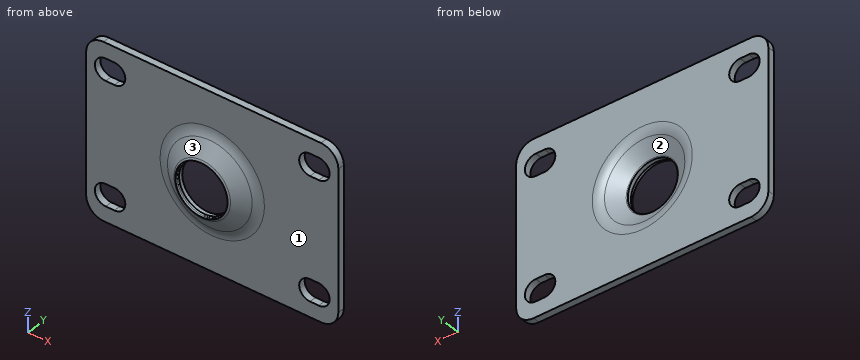
from build123d import *

# Parameters (mm, degrees)
SK_PLATE_OUTLINE_SLOTS_R = 19.05
EXT_PLATE_DEPTH          = 2.54


with BuildPart() as part:
    # Sk_pressed_centre → Rev_pressed_centre (revolve)
    with BuildSketch(Plane.XY, mode=Mode.PRIVATE) as rev_pressed_centre_sk:
        with BuildLine():
            Line((19.304, 69.85), (18.2626, 69.85))
            ThreePointArc((18.2626, 69.85), (16.381490046, 69.564975304), (14.669516, 68.73494))
            Line((14.669516, 68.73494), (9.54024, 65.2145))
            ThreePointArc((9.54024, 65.2145), (9.341458064, 65.091180356), (9.1313, 64.98844))
            Line((9.1313, 64.98844), (9.1313, 63.5508))
            Line((9.1313, 63.5508), (9.1567, 63.5508))
            ThreePointArc((9.1567, 63.5508), (9.426107684, 63.439207684), (9.5377, 63.1698))
            Line((9.5377, 63.1698), (9.5377, 62.31382))
            ThreePointArc((9.5377, 62.31382), (9.947965238, 62.460661275), (10.32764, 62.6745))
            Line((10.32764, 62.6745), (15.45717, 66.19494))
            ThreePointArc((15.45717, 66.19494), (17.169221611, 67.02429691), (19.05, 67.31))
            Line((19.05, 67.31), (19.304, 67.31))
            Line((19.304, 67.31), (19.304, 69.85))
        make_face()
    revolve(rev_pressed_centre_sk.sketch.rotate(Axis((0, -25.4, 0), (0, 1, 0)), 90), axis=Axis((0, -25.4, 0), (0, 1, 0)))

    # Sk_plate_outline_slots → Ext_plate (add)
    with BuildSketch(Plane(origin=(0, 67.31, 0), x_dir=(1, 0, 0), z_dir=(0, 1, 0))):
        with BuildLine():
            Line((-39.6875, 31.75), (39.6875, 31.75))
            ThreePointArc((39.6875, 31.75), (44.177628061, 29.890128061), (46.0375, 25.4))
            Line((46.0375, 25.4), (46.0375, -25.4))
            ThreePointArc((46.0375, -25.4), (44.177628061, -29.890128061), (39.6875, -31.75))
            Line((39.6875, -31.75), (-39.6875, -31.75))
            ThreePointArc((-39.6875, -31.75), (-44.177628061, -29.890128061), (-46.0375, -25.4))
            Line((-46.0375, -25.4), (-46.0375, 25.4))
            ThreePointArc((-46.0375, 25.4), (-44.177628061, 29.890128061), (-39.6875, 31.75))
        make_face()
        Circle(SK_PLATE_OUTLINE_SLOTS_R, mode=Mode.SUBTRACT)
        with BuildLine():
            Line((-38.89375, 26.19375), (-35.71875, 26.19375))
            ThreePointArc((-35.71875, 26.19375), (-31.75, 22.225), (-35.71875, 18.25625))
            Line((-35.71875, 18.25625), (-38.89375, 18.25625))
            ThreePointArc((-38.89375, 18.25625), (-42.8625, 22.225), (-38.89375, 26.19375))
        make_face(mode=Mode.SUBTRACT)
        with BuildLine():
            Line((-38.89375, -18.25625), (-35.71875, -18.25625))
            ThreePointArc((-35.71875, -18.25625), (-31.75, -22.225), (-35.71875, -26.19375))
            Line((-35.71875, -26.19375), (-38.89375, -26.19375))
            ThreePointArc((-38.89375, -26.19375), (-42.8625, -22.225), (-38.89375, -18.25625))
        make_face(mode=Mode.SUBTRACT)
        with BuildLine():
            Line((35.71875, 26.19375), (38.89375, 26.19375))
            ThreePointArc((38.89375, 26.19375), (42.8625, 22.225), (38.89375, 18.25625))
            Line((38.89375, 18.25625), (35.71875, 18.25625))
            ThreePointArc((35.71875, 18.25625), (31.75, 22.225), (35.71875, 26.19375))
        make_face(mode=Mode.SUBTRACT)
        with BuildLine():
            Line((35.71875, -18.25625), (38.89375, -18.25625))
            ThreePointArc((38.89375, -18.25625), (42.8625, -22.225), (38.89375, -26.19375))
            Line((38.89375, -26.19375), (35.71875, -26.19375))
            ThreePointArc((35.71875, -26.19375), (31.75, -22.225), (35.71875, -18.25625))
        make_face(mode=Mode.SUBTRACT)
    extrude(amount=EXT_PLATE_DEPTH)


solid = part.part
Source: CAD feature listing. Evaluate the final solid. Frame: model axes, mm. Face numbers are marked on the shaded views. Give positions to 0.01 mm unless a question says otherwise; leave off trailing zeros. Write each loop counter-clockwise with the first axis right and the second up, starting at its lowest first coordinate (ties: lowest second). Pieces come first, ordered by that corner, then holes. Notation, with made-up numbers: M 87,-32 L 140,-32 A19 ccw 140,-3 Z; hole C -29.5,84.25 d8. An arc over 180 degrees is marked long. Return JSON: item names as keys, results as strings. Group by question number.
1) Cut plane C-C, the plane x = 34. Output: boundary loops of the cut face in (y, z).
2) Draft query along X for the marked faces 1, 2 and 3. Return one class per face: released by +X, released by -X, zero draft, split by the parting line, or undercut.
3) Cut plane D-D, the plane z = 21. Output: boundary loops of the cut face in (x, y), then the cut area to 3 significant figures.
4) Ray query, L1, parallel to X at y = 69.5, z = -19; L2, parallel to Y at x = -30, z = -25. Return the intervals inside material, ascending.
5) First-contact query: pin 1 Ø21 at (x, z) = (0, 0) entering from +Y; pin 2 Ø4 at (x, z) = (36, -25) entering from -Y; pin 3 Ø11.5 at (x, z) = (0, 0) entering from +Y. Flat tips, straight axial feed; report the tip coordinate or a pass-through.
Data:
{
 "1": {"outline": "M 67.31,-31.75 L 69.85,-31.75 L 69.85,-25.8 L 67.31,-25.8 Z; M 67.31,-18.65 L 69.85,-18.65 L 69.85,18.65 L 67.31,18.65 Z; M 67.31,25.8 L 69.85,25.8 L 69.85,31.75 L 67.31,31.75 Z"},
 "2": {"face 1": "zero draft", "face 2": "undercut", "face 3": "split by the parting line"},
 "3": {"outline": "M -46.04,67.31 L -42.67,67.31 L -42.67,69.85 L -46.04,69.85 Z; M -31.94,67.31 L 31.94,67.31 L 31.94,69.85 L -31.94,69.85 Z; M 42.67,67.31 L 46.04,67.31 L 46.04,69.85 L 42.67,69.85 Z", "area": "179 mm²"},
 "4": {"L1": "x = -46.04 to -41.21, -33.41 to 33.41, 41.21 to 46.04", "L2": "y = 67.31 to 69.85"},
 "5": {"pin 1": "stops at y = 65.87", "pin 2": "stops at y = 67.31", "pin 3": "passes through"}
}
